Here's the drawing with two shaded views (mm, measured from the low corner). I have some questions. Round coordinates to 2 decimals unless told otherwise and drop trailing zeros. Order: outer loops, then holes, each group sorted by start corner. A loop starts at its lowest first (then second) coordinate and runs counter-clockwise, first axis right, second up. Notation, with made-up numbers: (89, 58) -> (141, 58) arc R27 cw to (141, 76) -> close; hole circle Ø1 at (9, 49). An arc over 180 degrees is marked (long way). Answer in a Markdown table with one row per item.
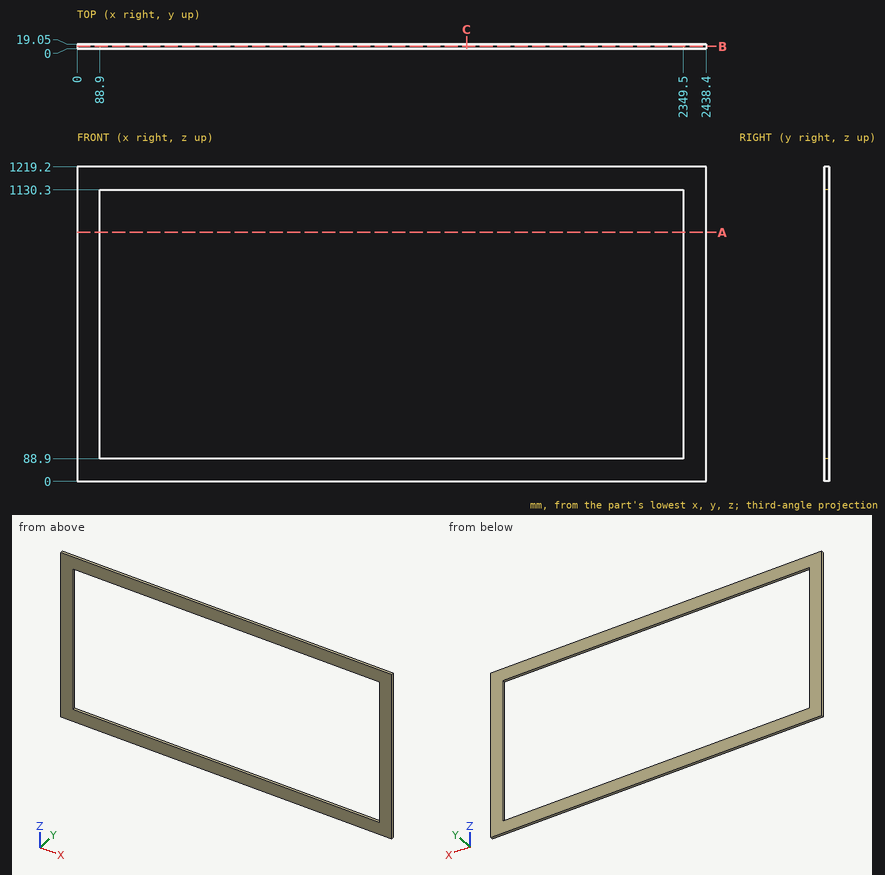
1. Please list where these lines run through material, in increasing order: line 1 along Z through (x, y) = (1562.5, 9); line 2 along X through (y, z) = (7, 103.5).
Numbers:
| item | result |
|---|---|
| line 1 | z = 0 to 88.9, 1130.3 to 1219.2 |
| line 2 | x = 0 to 88.9, 2349.5 to 2438.4 |
2. Suppose I cut it at A-A on z = 965. Write out the boundary of the cut face in (x, y), then the cut area to 3 significant figures.
Numbers:
| item | result |
|---|---|
| outline | (0, 0) -> (88.9, 0) -> (88.9, 19.05) -> (0, 19.05) -> close; (2349.5, 0) -> (2438.4, 0) -> (2438.4, 19.05) -> (2349.5, 19.05) -> close |
| area | 3,390 mm2 |
3. Suppose I cut it at C-C on x = 1510. Write out the boundary of the cut face in (y, z), then the cut area to 3 significant figures.
Numbers:
| item | result |
|---|---|
| outline | (0, 0) -> (19.05, 0) -> (19.05, 88.9) -> (0, 88.9) -> close; (0, 1130.3) -> (19.05, 1130.3) -> (19.05, 1219.2) -> (0, 1219.2) -> close |
| area | 3,390 mm2 |
4. Suppose I cut it at B-B on y = 10.25. Write out the boundary of the cut face in (x, z).
Numbers:
| item | result |
|---|---|
| outline | (0, 0) -> (2438.4, 0) -> (2438.4, 1219.2) -> (0, 1219.2) -> close; hole (88.9, 88.9) -> (2349.5, 88.9) -> (2349.5, 1130.3) -> (88.9, 1130.3) -> close |
